from build123d import *

# Parameters (mm, degrees)
SKETCH1_R            = 50
BOSS_EXTRUDE1_DEPTH  = 10
SKETCH2_R            = 15
CUT_EXTRUDE1_DEPTH   = 10
SKETCH3_R            = 60
BOSS_EXTRUDE2_DEPTH  = 10
SKETCH4_W            = 86.5466222
SKETCH4_H            = 83.124498108
BOSS_EXTRUDE3_DEPTH  = 40
BOSS_EXTRUDE9_DEPTH  = 83.124498108
SKETCH16_W           = 40
SKETCH16_H           = 180
CUT_EXTRUDE6_DEPTH   = 1000
SKETCH17_R           = 15
BOSS_EXTRUDE10_DEPTH = 61.562249054


with BuildPart() as part:
    # Sketch1 → Boss-Extrude1 (new body)
    with BuildSketch(Plane(origin=(0, 0, 0), x_dir=(1, 0, 0), z_dir=(0, 1, 0))):
        with Locations(Location((0, 0, 0), (0, 0, 270))):
            Circle(SKETCH1_R)
    extrude(amount=BOSS_EXTRUDE1_DEPTH)

    # Sketch2 → Cut-Extrude1 (cut)
    with BuildSketch(Plane(origin=(0, 10, 0), x_dir=(1, 0, 0), z_dir=(0, 1, 0))):
        with Locations(Location((0, 0, 0), (0, 0, 270))):
            Circle(SKETCH2_R)
    extrude(amount=-CUT_EXTRUDE1_DEPTH, mode=Mode.SUBTRACT)

    # Sketch3 → Boss-Extrude2 (add)
    with BuildSketch(Plane(origin=(0, 10, 0), x_dir=(1, 0, 0), z_dir=(0, 1, 0))):
        with Locations(Location((0, 0, 0), (0, 0, 270))):
            Circle(SKETCH3_R)
    extrude(amount=BOSS_EXTRUDE2_DEPTH)

    # Sketch4 → Boss-Extrude3 (add)
    with BuildSketch(Plane(origin=(0, 20, 0), x_dir=(1, 0, 0), z_dir=(0, 1, 0))):
        Rectangle(SKETCH4_W, SKETCH4_H)
    extrude(amount=BOSS_EXTRUDE3_DEPTH)

    # Sketch15 → Boss-Extrude9 (add)
    with BuildSketch(Plane.XY.offset(41.562249054)):
        with BuildLine():
            Line((-40, 60), (-40, 150))
            ThreePointArc((-40, 150), (0, 190), (40, 150))
            Line((40, 150), (40, 60))
            ThreePointArc((40, 60), (0, 20), (-40, 60))
        make_face()
    extrude(amount=-BOSS_EXTRUDE9_DEPTH)

    # Sketch16 → Cut-Extrude6 (cut)
    with BuildSketch(Plane.ZY.offset(40)):
        with Locations((0, 150)):
            Rectangle(SKETCH16_W, SKETCH16_H)
    extrude(amount=-CUT_EXTRUDE6_DEPTH, mode=Mode.SUBTRACT)

    # Sketch17 → Boss-Extrude10 (add)
    with BuildSketch(Plane.XY.offset(41.562249054)):
        with Locations((0, 150)):
            Circle(SKETCH17_R)
    extrude(amount=-BOSS_EXTRUDE10_DEPTH)


solid = part.part
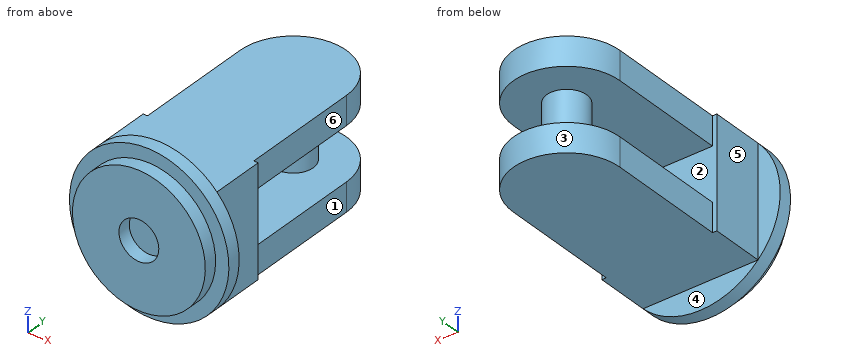
Part model, mm, in its own coordinate system. Face numbers are marked on the shaded views. A direction names the side the tool comes from. Round coordinates to 2 decimals unless told otherwise and drop trailing zeros. Loops run counter-clockwise (first coordinate to the right, second up) from the corner with the lowest first, then second, coordinate; pieces in that order, holes last. Notation, with made-up numbers: (-23, 77) - (13, 77) arc R29 cw to (13, 99) - close; hole circle Ø5 at (10.5, 74). An arc over 180 degrees is marked (long way). Answer as a JSON object with one key per item and string values.
Item 1: Pin check, flat tips, straight feed: pin 1 (9 mm diameter, centred on x = -9, z = 48, fed in from +Y); pin 2 (23.5 mm diameter, centred on y = 99, z = 28, fed in from -X); pin 3 (9 mm diameter, centred on x = 0.5, z = -7.5, fed in from -Y); pin 4 (1 mm diameter, centred on y = 156.5, z = 42.5, fed in from +X). Stop position of each tip, or through.
Output:
{"pin 1": "y = 20", "pin 2": "x = -40", "pin 3": "y = 10", "pin 4": "through"}
Item 2: Tool access for the marked faces 4, 5 and 6: list every direction of +Z, -Z, +X, -X, +Y, -Y with a clear straight run to the whole face (end or side of a thin tool).
Output:
{"face 4": "-Z, +X, -X, +Y", "face 5": "+Z, -Z, -X, +Y", "face 6": "+Z, -Z, +X, +Y"}
Item 3: Band-saw the part on A-A on z = 0. List the corners of the cut face in (x, y).
Output:
{"outline": "(-60, 10) - (-50, 10) - (-50, 0) - (-15, 0) - (-15, 10) - (15, 10) - (15, 0) - (50, 0) - (50, 10) - (60, 10) - (60, 20) - (43.27, 20) - (43.27, 60) - (-43.27, 60) - (-43.27, 20) - (-60, 20) - close; circle Ø30 at (0, 150)"}
Item 4: Pull direction Y, two halves, no side cores. Call the marked faces 1, 2 and 3: pulls with the +Y half, pulls with the -Y half, needs draft (parallel to the pull), parting line crosses it, or undercut.
Output:
{"face 1": "needs draft", "face 2": "undercut", "face 3": "pulls with the +Y half"}
Item 5: Band-saw the part on B-B on y = 121.5. List the corners of the cut face in (x, z), plus the area to 3 significant figures.
Output:
{"outline": "(-40, -41.56) - (40, -41.56) - (40, -20) - (-40, -20) - close; (-40, 20) - (40, 20) - (40, 41.56) - (-40, 41.56) - close", "area": "3,450 mm2"}
Item 6: Band-saw the part on D-D on x = -19.5. List the corners of the cut face in (y, z), plus the area to 3 significant figures.
Output:
{"outline": "(0, -46.04) - (10, -46.04) - (10, -56.74) - (20, -56.74) - (20, -41.56) - (184.92, -41.56) - (184.92, -20) - (60, -20) - (60, 20) - (184.92, 20) - (184.92, 41.56) - (20, 41.56) - (20, 56.74) - (10, 56.74) - (10, 46.04) - (0, 46.04) - close", "area": "10,800 mm2"}
Item 7: Band-saw the part on C-C on x = 0. List the corners of the cut face in (y, z).
Output:
{"outline": "(0, -50) - (10, -50) - (10, -60) - (20, -60) - (20, -41.56) - (190, -41.56) - (190, -20) - (165, -20) - (165, 20) - (190, 20) - (190, 41.56) - (20, 41.56) - (20, 60) - (10, 60) - (10, 50) - (0, 50) - (0, 15) - (10, 15) - (10, -15) - (0, -15) - close; hole (60, -20) - (135, -20) - (135, 20) - (60, 20) - close"}
Item 8: Wall check: L1, parallel to X at y = 2, z = 0; L2, parallel to Y at x = -19, z = -2.5; L3, parallel to Y at x = 23, z = -44. Give the ranges that are in metal, low to high.
Output:
{"L1": "-50 to -15, 15 to 50", "L2": "0 to 60", "L3": "0 to 20"}
